Verification items for the finished model (mm, model axes). Face numbers are marked on the shaded views. A direction names the side the tool comes from. Give positions to 0.01 mm unless a question says otherwise; leave off trailing zeros. Order: outer loops, then holes, each group sorted by start corner. A loop starts at its lowest first (then second) coordinate and runs counter-clockwise, first axis right, second up.
(1) Sectioned sample at B-B on x = -7. Record the cut outline in (y, z), plus the area to 3 significant figures.
(2) Mould release check, pull along X, two halves, no side actions. Record for the marked faces 3, 4 and 5: pulls with the +X half, pulls with the -X half, needs draft (parallel to the pull), parting line crosses it, or undercut.
(3) Gauge pin test, flat ends, axial feed: pin 1 (7.5 mm diameter, centred on y = -17.5, z = 6.5, fed in from +X); pin 2 (1 mm diameter, centred on y = 9.5, z = 13, fed in from +X); pin 3 (8 mm diameter, centred on x = 15, z = 4.5, fed in from +Y). Record the tip position at first contact, or that the pin passes through.
(4) Sectioned sample at C-C on y = -17. Record the cut outline in (x, z) (3 decimals), plus the area to 3 significant figures.
(5) Access from +Z, -Z, +X, -X, +Y, -Y to the whole of each face (thin tool, end or side, straight path). Record for the marked faces 1 and 2.
(6) Scan lines: L1, parallel to Y at x = 0.5, z = 20.25; L2, parallel to X at y = -17, z = 5; L3, parallel to Y at x = -5, z = 5. Record each from-to range of solid material in increasing order.
(7) Sectioned sample at D-D on y = -11.5. Record the cut outline in (x, z), plus the area to 3 significant figures.
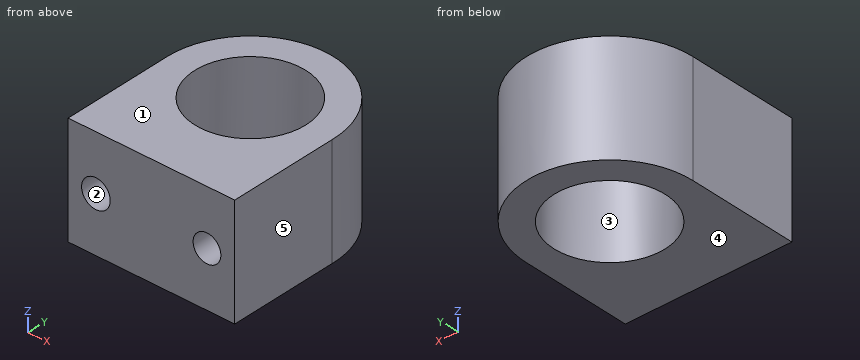
```python
from build123d import *

# Parameters (mm, degrees)
F0_R     = 12.7
F1_DEPTH = 25.4
F2_R     = 3.2766
F2_R_2   = 3.175
F3_DEPTH = 12.7


with BuildPart() as f1:
    # F0 (on Top) → F1 (new body)
    with BuildSketch(Plane.XY):
        with BuildLine():
            Line((19.048172, -25.4), (19.048172, -0.373213))
            ThreePointArc((19.048172, -0.373213), (0.186616, 19.050914), (-19.051828, 0))
            Line((-19.051828, 0), (-19.051828, -25.4))
            Line((-19.051828, -25.4), (19.048172, -25.4))
        make_face()
        Circle(F0_R, mode=Mode.SUBTRACT)
    extrude(amount=F1_DEPTH)

    # F2 (on face) → F3 (cut)
    with BuildSketch(Plane.XZ.offset(25.4)):
        with Locations((-12.701828, 12.7)):
            Circle(F2_R)
        with Locations((12.698172, 12.7)):
            Circle(F2_R_2)
    extrude(amount=-F3_DEPTH, mode=Mode.SUBTRACT)


solid = f1.part
```
Ans:
1. outline: (-25.4, 0) - (-10.6, 0) - (-10.6, 25.4) - (-25.4, 25.4) - close; (10.6, 0) - (17.72, 0) - (17.72, 25.4) - (10.6, 25.4) - close
1. area: 557 mm2
2. face 3: undercut
2. face 4: needs draft
2. face 5: pulls with the +X half
3. pin 1: stops at x = 19.05
3. pin 2: stops at x = 16.79
3. pin 3: stops at y = 15.56
4. outline: (-19.052, 0) - (19.048, 0) - (19.048, 25.4) - (-19.052, 25.4) - close; hole circle Ø6.553 at (-12.702, 12.7); hole circle Ø6.35 at (12.698, 12.7)
4. area: 902 mm2
5. face 1: +Z, +X, -X, +Y, -Y
5. face 2: -Y
6. L1: y = -25.4 to -12.69, 12.69 to 19.05
6. L2: x = -19.05 to 19.05
6. L3: y = -25.4 to -11.67, 11.67 to 18.38
7. outline: (-19.05, 0) - (-5.39, 0) - (-5.39, 25.4) - (-19.05, 25.4) - close; (5.39, 0) - (19.05, 0) - (19.05, 25.4) - (5.39, 25.4) - close
7. area: 694 mm2
